from build123d import *

# Parameters (mm, degrees)
SKETCH1_W                               = 304.8
SKETCH1_H                               = 304.8
BOSS_EXTRUDE1_DEPTH                     = 28.575
SKETCH2_R                               = 6.5151
HAAS_T_SLOT_HOLES_DEPTH                 = 218.41216761
SKETCH3_R                               = 9.779
HAAS_COUNTER_BORES_DEPTH                = 19.05
SKETCH4_R                               = 6.5151
TORMACH_T_SLOT_HOLES_DEPTH              = 218.41216761
SKETCH5_R                               = 9.779
TORMACH_COUNTER_BORES_DEPTH             = 19.05
SKETCH6_R                               = 2.99974
SPROCKET_LOCATING_HOLES_DEPTH           = 19.05
SKETCH7_R                               = 2.99974
SPROCKET_MOUNTING_CLEARANCE_HOLES_DEPTH = 19.05
SKETCH8_R                               = 5.9182
F_1_2_13_TAPPED_HOLES_DEPTH             = 19.05
SKETCH9_R                               = 3.175
F_1_4_20_SPROCKET_FIXTURE_BOLTS_DEPTH   = 19.05


with BuildPart() as part:
    # Sketch1 → Boss-Extrude1 (new body)
    with BuildSketch(Plane.XY):
        Rectangle(SKETCH1_W, SKETCH1_H)
    extrude(amount=BOSS_EXTRUDE1_DEPTH)

    # Sketch2 → HAAS T-Slot Holes (cut, through all)
    with BuildSketch(Plane.XY.offset(28.575)):
        with Locations((-127, 101.6)):
            Circle(SKETCH2_R)
        with Locations((127, 101.6)):
            Circle(SKETCH2_R)
        with Locations((127, -101.6)):
            Circle(SKETCH2_R)
        with Locations((-127, -101.6)):
            Circle(SKETCH2_R)
        Circle(SKETCH2_R)
    extrude(amount=-HAAS_T_SLOT_HOLES_DEPTH, mode=Mode.SUBTRACT)

    # Sketch3 → HAAS Counter Bores (cut)
    with BuildSketch(Plane.XY.offset(28.575)):
        with Locations((-127, 101.6)):
            Circle(SKETCH3_R)
        with Locations((127, 101.6)):
            Circle(SKETCH3_R)
        Circle(SKETCH3_R)
        with Locations((127, -101.6)):
            Circle(SKETCH3_R)
        with Locations((-127, -101.6)):
            Circle(SKETCH3_R)
    extrude(amount=-HAAS_COUNTER_BORES_DEPTH, mode=Mode.SUBTRACT)

    # Sketch4 → Tormach T-Slot Holes (cut, through all)
    with BuildSketch(Plane.XY.offset(28.575)):
        with Locations((-101.6, 90.4875)):
            Circle(SKETCH4_R)
        with Locations((101.6, 90.4875)):
            Circle(SKETCH4_R)
        with Locations((-101.6, -90.4875)):
            Circle(SKETCH4_R)
        with Locations((101.6, -90.4875)):
            Circle(SKETCH4_R)
    extrude(amount=-TORMACH_T_SLOT_HOLES_DEPTH, mode=Mode.SUBTRACT)

    # Sketch5 → Tormach Counter bores (cut)
    with BuildSketch(Plane.XY.offset(28.575)):
        with Locations((-101.6, 90.4875)):
            Circle(SKETCH5_R)
        with Locations((101.6, 90.4875)):
            Circle(SKETCH5_R)
        with Locations((101.6, -90.4875)):
            Circle(SKETCH5_R)
        with Locations((-101.6, -90.4875)):
            Circle(SKETCH5_R)
    extrude(amount=-TORMACH_COUNTER_BORES_DEPTH, mode=Mode.SUBTRACT)

    # Sketch6 → Sprocket Locating Holes (cut)
    with BuildSketch(Plane.XY.offset(28.575)):
        with Locations((0, 43.50004)):
            Circle(SKETCH6_R)
        with Locations((0, -43.50004)):
            Circle(SKETCH6_R)
    extrude(amount=-SPROCKET_LOCATING_HOLES_DEPTH, mode=Mode.SUBTRACT)

    # Sketch7 → Sprocket Mounting clearance holes (cut)
    with BuildSketch(Plane.XY.offset(28.575)):
        with Locations((43.50004, 0)):
            Circle(SKETCH7_R)
        with Locations((37.672139706, -21.75002)):
            Circle(SKETCH7_R)
        with Locations((21.75002, -37.672139706)):
            Circle(SKETCH7_R)
        with Locations((-21.75002, -37.672139706)):
            Circle(SKETCH7_R)
        with Locations((-37.672139706, -21.75002)):
            Circle(SKETCH7_R)
        with Locations((-43.50004, 0)):
            Circle(SKETCH7_R)
        with Locations((-37.672139706, 21.75002)):
            Circle(SKETCH7_R)
        with Locations((-21.75002, 37.672139706)):
            Circle(SKETCH7_R)
        with Locations((21.75002, 37.672139706)):
            Circle(SKETCH7_R)
        with Locations((37.672139706, 21.75002)):
            Circle(SKETCH7_R)
    extrude(amount=-SPROCKET_MOUNTING_CLEARANCE_HOLES_DEPTH, mode=Mode.SUBTRACT)

    # Sketch8 → 1/2-13 Tapped Holes (cut)
    with BuildSketch(Plane.XY.offset(28.575)):
        with Locations((-71.4375, 106.4641)):
            Circle(SKETCH8_R)
        with Locations((71.4375, 106.4641)):
            Circle(SKETCH8_R)
        with Locations((71.4375, -106.4641)):
            Circle(SKETCH8_R)
        with Locations((-71.4375, -106.4641)):
            Circle(SKETCH8_R)
    extrude(amount=-F_1_2_13_TAPPED_HOLES_DEPTH, mode=Mode.SUBTRACT)

    # Sketch9 → 1/4-20 Sprocket Fixture Bolts (cut)
    with BuildSketch(Plane.XY.offset(28.575)):
        with Locations((0, 62.865)):
            Circle(SKETCH9_R)
        with Locations((31.4325, 54.442687009)):
            Circle(SKETCH9_R)
        with Locations((54.442687009, 31.4325)):
            Circle(SKETCH9_R)
        with Locations((62.865, 0)):
            Circle(SKETCH9_R)
        with Locations((54.442687009, -31.4325)):
            Circle(SKETCH9_R)
        with Locations((31.4325, -54.442687009)):
            Circle(SKETCH9_R)
        with Locations((0, -62.865)):
            Circle(SKETCH9_R)
        with Locations((-31.4325, -54.442687009)):
            Circle(SKETCH9_R)
        with Locations((-54.442687009, -31.4325)):
            Circle(SKETCH9_R)
        with Locations((-62.865, 0)):
            Circle(SKETCH9_R)
        with Locations((-54.442687009, 31.4325)):
            Circle(SKETCH9_R)
        with Locations((-31.4325, 54.442687009)):
            Circle(SKETCH9_R)
    extrude(amount=-F_1_4_20_SPROCKET_FIXTURE_BOLTS_DEPTH, mode=Mode.SUBTRACT)


solid = part.part
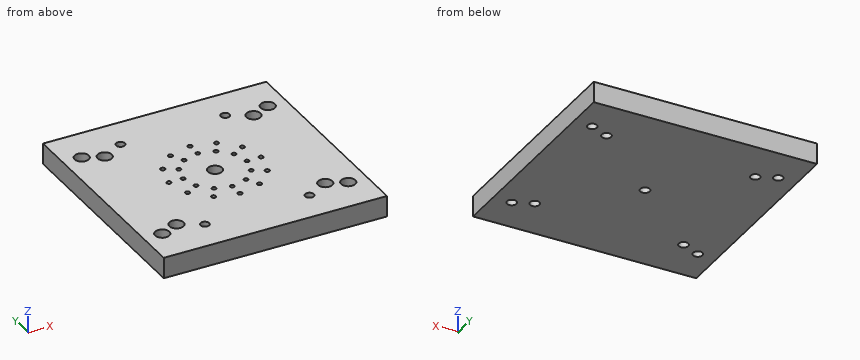
Verification items for the finished model (mm, model axes). Coordinates: 2 decimals unless noted, no trailing zeros. Order: outer loops, then holes, each group sorted by start corner. A loop starts at its lowest first (then second) coordinate and runs counter-clockwise, first axis right, second up.
1. Go/stop test with a flat-tipped pin: pin 1 Ø6 at (x, y) = (-73, -104.5) entering from +Z (3 decimals). Record where the tip stops, or that it passes through.
Results found:
pin 1: stops at z = 9.525
2. Sectioned sample at A-A, the plane x = -127. Record the cut outline in (y, z) (3 decimals), and give its area (3 significant figures).
Results found:
outline: (-152.4, 0) - (-108.115, 0) - (-108.115, 9.525) - (-111.379, 9.525) - (-111.379, 28.575) - (-152.4, 28.575) - close; (-95.085, 0) - (95.085, 0) - (95.085, 9.525) - (91.821, 9.525) - (91.821, 28.575) - (-91.821, 28.575) - (-91.821, 9.525) - (-95.085, 9.525) - close; (108.115, 0) - (152.4, 0) - (152.4, 28.575) - (111.379, 28.575) - (111.379, 9.525) - (108.115, 9.525) - close
area: 7,720 mm2
3. Scan lines: line 1 (Y direction, x = 127, z = 4); line 2 (Y direction, x = 101.6, z = 16); line 3 (Y direction, x = 0, z = 14). Record each from-to range of solid material in increasing order.
Results found:
line 1: y = -152.4 to -108.12, -95.08 to 95.08, 108.12 to 152.4
line 2: y = -152.4 to -100.27, -80.71 to 80.71, 100.27 to 152.4
line 3: y = -152.4 to -66.04, -59.69 to -46.5, -40.5 to -9.78, 9.78 to 40.5, 46.5 to 59.69, 66.04 to 152.4
4. Sectioned sample at B-B, the plane x = 70. Record the cut outline in (y, z) (3 decimals).
Results found:
outline: (-152.4, 0) - (152.4, 0) - (152.4, 28.575) - (112.205, 28.575) - (112.205, 9.525) - (100.723, 9.525) - (100.723, 28.575) - (-100.723, 28.575) - (-100.723, 9.525) - (-112.205, 9.525) - (-112.205, 28.575) - (-152.4, 28.575) - close
5. Sectioned sample at C-C, the plane z = 15.25. Give the number of separate pieces and of enclosed holes in the cut face, and give its area (3 significant figures).
Results found:
separate pieces: 1
enclosed holes: 37
area: 89,000 mm2
